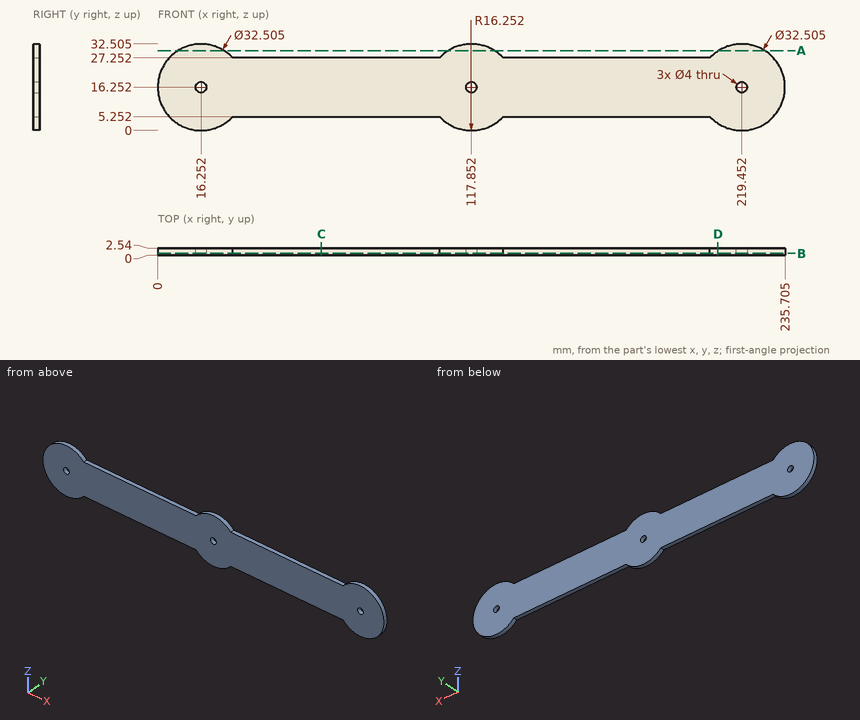
Input: dimensioned drawing with shaded views. Units: mm. Origin: part minimum x, y, z. Round coordinates to 2 decimals unless told otherwise and drop trailing zeros. Loops run counter-clockwise (first coordinate to the right, second up) from the corner with the lowest first, then second, coordinate; pieces in that order, holes last. Notation, with made-up numbers: (40.5, 75) -> (59.5, 75) arc R34 ccw to (59.5, 107) -> close; hole circle Ø9 at (43, 66.5). An arc over 180 degrees is marked (long way). Use one line per item in the form item = value. Start each with the question number.
1) Section B-B on y = 0.7. Output: boundary loops of the cut face in (x, z) (1 decimal).
2) First-contact query: P1, Ø1.5, axis at x = 47.5, y = 1, coming from the -Z side; P2, Ø3.5, axis at x = 117.85, z = 16.25, coming from the +Y side; P3, Ø0.8, axis at x = 81.5, y = 1, coming from the +Z side. Flat tips, straight axial feed; report the tip coordinate or a pass-through.
3) Section A-A on z = 30. Output: boundary loops of the cut face in (x, y).
4) Section C-C on x = 61.5. Output: boundary loops of the cut face in (y, z).
5) Line query: L1, parallel to X at y = 1.25, z = 16.5; L2, parallel to X at y = 0.55, z = 15.5 (1 decimal); L3, parallel to X at y = 2.1, z = 2 (1 decimal). Output: solid intervals per line, ascending.
6) Section D-D on x = 210.5. Output: boundary loops of the cut face in (y, z).
Response:
q1.outline = (28.2, 5.3) -> (105.9, 5.3) arc R16.3 ccw to (129.8, 5.3) -> (207.5, 5.3) arc R16.3 ccw (long way) to (207.5, 27.3) -> (129.8, 27.3) arc R16.3 ccw to (105.9, 27.3) -> (28.2, 27.3) arc R16.3 ccw (long way) to start; hole circle Ø4 at (16.3, 16.3); hole circle Ø4 at (117.9, 16.3); hole circle Ø4 at (219.5, 16.3)
q2.P1 = 5.25
q2.P2 = through
q2.P3 = 27.25
q3.outline = (7.58, 0) -> (24.92, 0) -> (24.92, 2.54) -> (7.58, 2.54) -> close; (109.18, 0) -> (126.52, 0) -> (126.52, 2.54) -> (109.18, 2.54) -> close; (210.78, 0) -> (228.12, 0) -> (228.12, 2.54) -> (210.78, 2.54) -> close
q4.outline = (0, 5.25) -> (2.54, 5.25) -> (2.54, 27.25) -> (0, 27.25) -> close
q5.L1 = 0 to 14.27, 18.24 to 115.87, 119.84 to 217.47, 221.44 to 235.7
q5.L2 = 0 to 14.4, 18.1 to 116, 119.7 to 217.6, 221.3 to 235.7
q5.L3 = 8.4 to 24.1, 110 to 125.7, 211.6 to 227.3
q6.outline = (0, 2.69) -> (2.54, 2.69) -> (2.54, 29.82) -> (0, 29.82) -> close
